```python
from build123d import *

# Parameters (mm, degrees)
EXTRUDE_1_DEPTH     = 3
SKETCH_2_R          = 1.55
CUT_EXTRUDE_1_DEPTH = 24.464866076


with BuildPart() as part:
    # 草图1 → 凸台-拉伸1 (new body)
    with BuildSketch(Plane(origin=(0, 0, 0), x_dir=(1, 0, 0), z_dir=(0, 1, 0))):
        with BuildLine():
            Line((-10.5, 8), (-10.5, -8))
            ThreePointArc((-10.5, -8), (-11.796148944, -7.89430161), (-13.058047675, -7.579999479))
            ThreePointArc((-13.058047675, -7.579999479), (-20.257809372, -7.8125), (-18.455991924, -0.837969271))
            ThreePointArc((-18.455991924, -0.837969271), (-18.5, 0), (-18.455991924, 0.837969271))
            ThreePointArc((-18.455991924, 0.837969271), (-20.257809372, 7.8125), (-13.058047675, 7.579999479))
            ThreePointArc((-13.058047675, 7.579999479), (-11.796148944, 7.89430161), (-10.5, 8))
        make_face()
    extrude(amount=EXTRUDE_1_DEPTH)

    # 草图2 → 切除-拉伸1 (cut, through all)
    with BuildSketch(Plane(origin=(0, 3, 0), x_dir=(1, 0, 0), z_dir=(0, 1, 0))):
        with Locations(Location((-17.681747698, 5.75, 0), (0, 0, 270))):
            Circle(SKETCH_2_R)
        with Locations(Location((-17.681747698, -5.75, 0), (0, 0, 270))):
            Circle(SKETCH_2_R)
    extrude(amount=-CUT_EXTRUDE_1_DEPTH, mode=Mode.SUBTRACT)


solid = part.part
```
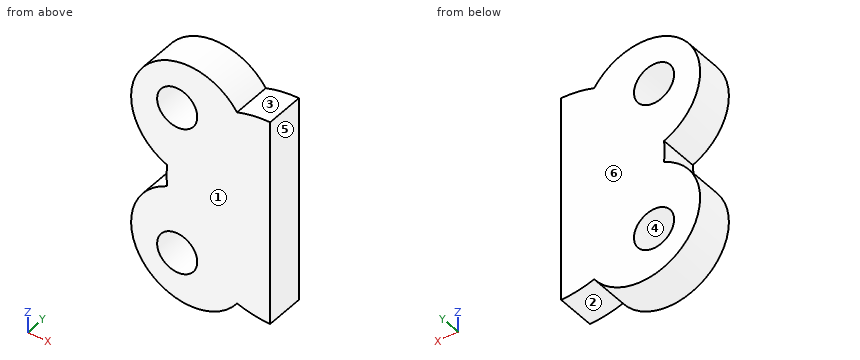
For this review, take the finished solid that the model builds, in its own axes (mm). Face numbers are marked on the shaded views. A direction names the side the tool comes from. Coordinates: 2 decimals unless noted, no trailing zeros. Loops run counter-clockwise (first coordinate to the right, second up) from the corner with the lowest first, then second, coordinate; pieces in that order, holes last. Notation, with made-up numbers: (43.5, -34) -> (97.5, -34) arc R27 cw to (97.5, -2) -> close; hole circle Ø9 at (-4, 60). An arc over 180 degrees is marked (long way). Return JSON: item names as keys, results as strings. Group by question number.
(1) Consider section A-A, the plane z = -4.5. Give the boundary of the cut face in (x, y).
(2) To check wall thickness, follow L1, parallel to Z at x = -17.5, y = 1.25; L2, parallel to X at y = 2.4, z = -5.75; L3, parallel to Z at x = -18.75, y = 1.6. State the ranges of each line that lie inside material, in increasing order.
(3) Consider section C-C, the plane x = -18.25. Give the boundary of the cut face in (y, z).
(4) Mouldability with a two-part tool opening along X and no side actions: class the marked faces 4, 5 and 6 as pulls with the +X half, pulls with the -X half, needs draft (parallel to the pull), parting line crosses it, or undercut.
(5) Tool access review of the marked faces 1, 2 and 3: name each direction out of +Z, -Z, +X, -X, +Y, -Y from which nothing blocks a thin tool from reaching the whole face with its end or side.
(6) Consider section B-B, the plane x = -20. Give the boundary of the cut face in (y, z).
(7) Consider section D-D, the plane y = 0.65. Give the boundary of the cut face in (x, z) (3 decimals).
Results below:
{
 "1": {"outline": "(-21.22, 0) -> (-18.6, 0) -> (-18.6, 3) -> (-21.22, 3) -> close; (-16.77, 0) -> (-10.5, 0) -> (-10.5, 3) -> (-16.77, 3) -> close"},
 "2": {"L1": "z = -9.44 to -7.29, -4.21 to 4.21, 7.29 to 9.44", "L2": "x = -21.18 to -19.23, -16.13 to -10.5", "L3": "z = -9.03 to -6.87, -4.63 to -0.97, 0.97 to 4.63, 6.87 to 9.03"},
 "3": {"outline": "(0, -9.24) -> (3, -9.24) -> (3, -7.19) -> (0, -7.19) -> close; (0, -4.31) -> (3, -4.31) -> (3, 4.31) -> (0, 4.31) -> close; (0, 7.19) -> (3, 7.19) -> (3, 9.24) -> (0, 9.24) -> close"},
 "4": {"face 4": "undercut", "face 5": "pulls with the +X half", "face 6": "needs draft"},
 "5": {"face 1": "+Z, -Z, +X, -X, -Y", "face 2": "-Z, +Y, -Y", "face 3": "+Z, +Y, -Y"},
 "6": {"outline": "(0, -8.11) -> (3, -8.11) -> (3, -1.89) -> (0, -1.89) -> close; (0, 1.89) -> (3, 1.89) -> (3, 8.11) -> (0, 8.11) -> close"},
 "7": {"outline": "(-18.456, -0.838) arc R4.5 ccw (long way) to (-13.058, -7.58) arc R8 ccw to (-10.5, -8) -> (-10.5, 8) arc R8 ccw to (-13.058, 7.58) arc R4.5 ccw (long way) to (-18.456, 0.838) arc R8 ccw to start; hole circle Ø3.1 at (-17.682, -5.75); hole circle Ø3.1 at (-17.682, 5.75)"}
}
